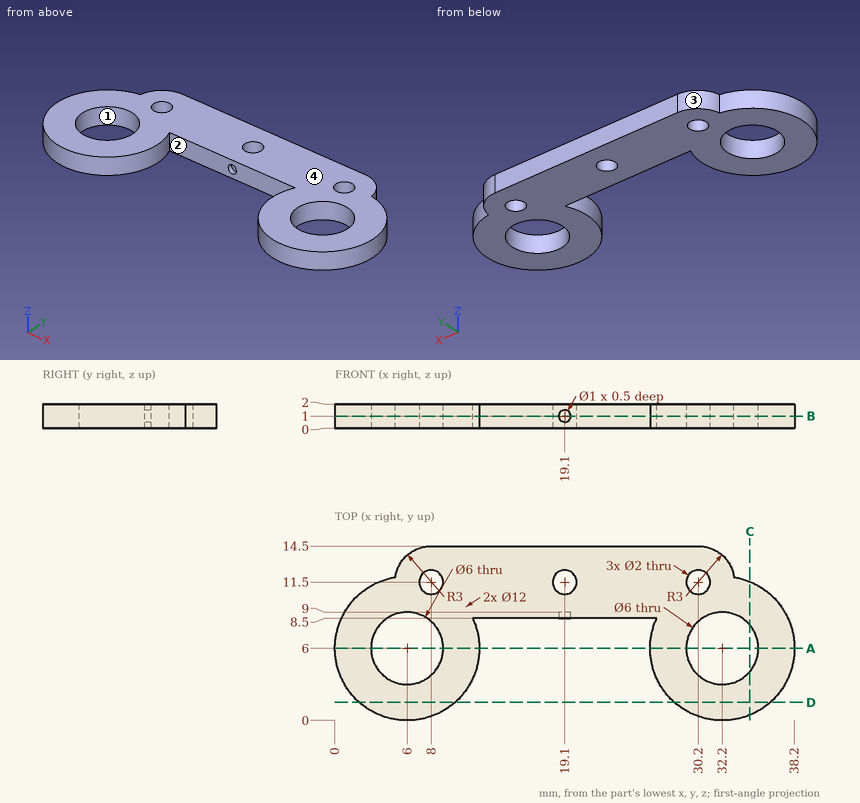
Geometry: see drawing. Coordinates: mm, zero at the bounding-box minimum. Coordinates: 2 decimals unless noted, no trailing zeros. Loops run counter-clockwise (first coordinate to the right, second up) from the corner with the lowest first, then second, coordinate; pieces in that order, holes last. Notation, with made-up numbers: (52, -34) -> (91, -34) arc R24 ccw to (91, -21) -> close; hole circle Ø9 at (67.5, 73.25). An arc over 180 degrees is marked (long way). Use a Markdown table: item, result.
1) Cut plane D-D (y = 1.5). Return the cut outline in (x, z).
Results found:
| item | result |
|---|---|
| outline | (2.03, 0) -> (9.97, 0) -> (9.97, 2) -> (2.03, 2) -> close; (28.23, 0) -> (36.17, 0) -> (36.17, 2) -> (28.23, 2) -> close |
2) Material intervals for line 1 along X through (y, z) = (6, 1.05); line 2 along X through (y, z) = (7, 1.6) (1 decimal); line 3 along Y through (x, z) = (6, 1.15) (1 decimal), sorted ascending. Write a range as from..to.
Results found:
| item | result |
|---|---|
| line 1 | x = 0..3, 9..12, 26.2..29.2, 35.2..38.2 |
| line 2 | x = 0.1..3.2, 8.8..11.9, 26.3..29.4, 35..38.1 |
| line 3 | y = 0..3, 9..13.7 |
3) Pull-direction query (X, two-part tool) for the marked faces 1, 2, 3 and 4; classes: released by +X, released by -X, zero draft, split by the parting line, or undercut.
Results found:
| item | result |
|---|---|
| face 1 | undercut |
| face 2 | undercut |
| face 3 | released by -X |
| face 4 | zero draft |
4) Cut plane A-A (y = 6). Return the cut outline in (x, z), then the cut area to 3 significant figures.
Results found:
| item | result |
|---|---|
| outline | (0, 0) -> (3, 0) -> (3, 2) -> (0, 2) -> close; (9, 0) -> (12, 0) -> (12, 2) -> (9, 2) -> close; (26.2, 0) -> (29.2, 0) -> (29.2, 2) -> (26.2, 2) -> close; (35.2, 0) -> (38.2, 0) -> (38.2, 2) -> (35.2, 2) -> close |
| area | 24.0 mm2 |
5) Cut plane C-C (x = 34.5). Return the cut outline in (y, z).
Results found:
| item | result |
|---|---|
| outline | (0.46, 0) -> (4.07, 0) -> (4.07, 2) -> (0.46, 2) -> close; (7.93, 0) -> (11.54, 0) -> (11.54, 2) -> (7.93, 2) -> close |
6) Contact query for flat-ended pins moving along their axis: pin 1 (5 mm diameter, centred on x = 6, y = 6, fed in from +Z); pin 2 (1 mm diameter, centred on y = 8, z = 1, fed in from +X); pin 3 (0.5 mm diameter, centred on x = 19.5, z = 1, fed in from -Y). Output: stop coordinate, or through.
Results found:
| item | result |
|---|---|
| pin 1 | passes through |
| pin 2 | stops at x = 38.01 |
| pin 3 | stops at y = 8.5 |
7) Cut plane B-B (z = 1). Return the cut outline in (x, y) (1 decimal).
Results found:
| item | result |
|---|---|
| outline | (5, 11.9) arc R6 ccw (long way) to (11.5, 8.5) -> (18.6, 8.5) -> (18.6, 9) -> (19.6, 9) -> (19.6, 8.5) -> (26.7, 8.5) arc R6 ccw (long way) to (33.2, 11.9) arc R3 ccw to (30.2, 14.5) -> (8, 14.5) arc R3 ccw to start; hole circle Ø6 at (6, 6); hole circle Ø2 at (8, 11.5); hole circle Ø2 at (19.1, 11.5); hole circle Ø6 at (32.2, 6); hole circle Ø2 at (30.2, 11.5) |
